Part model, mm, in its own coordinate system. A direction names the side the tool comes from. Coordinates: 2 decimals unless noted, no trailing zeros. Loops run counter-clockwise (first coordinate to the right, second up) from the corner with the lowest first, then second, coordinate; pieces in that order, holes last. Notation, with made-up numbers: M 60,8 L 82,8 A14 ccw 82,31 Z; hole C 78,45.25 d10. An arc over 180 degrees is marked long. Use a Markdown table: item, result. Add a question column.
1) Band-saw the part on A-A (z = 0.3). List the corners of the cut face in (x, y), plus the area to 3 significant figures.
2) Pull direction X, two halves, no side cores. Call faces 4 (the cylindrical face through (2, 3.7, 0.2)), 5 (the cylindrical face through (-6.048, 0.884, 0.85)), 6 (the cylindrical face through (-6.707, 0.627, 0.857)): released by +X, released by -X, zero draft, split by the parting line, or undercut.
3) Tool access for faces 1 (the cylindrical face through (1.95, 3.68, 0.86)), 2 (the cylindrical face through (-6.06, 0.88, 0.14)), 3 (the cylindrical face through (1.26, 3.53, 0.85)): list every direction of +Z, -Z, +X, -X, +Y, -Y with a clear straight run to the whole face (end or side of a thin tool).
4) Wall check: probe 1 along X at (y, z) = (14, 0.6); probe 2 along X at (y, z) = (-14, 0.15); probe 3 along Z at (x, y) = (-11.75, 21). Give the ranges that are in metal, low to high. Write a range as from..to.
Autodesk Inventor part; units mm, degrees
ref_plane "YZ Plane" through (0, 0, 0) normal (1, 0, 0) x (0, 1, 0)
ref_plane "XZ Plane" through (0, 0, 0) normal (0, 1, 0) x (-1, 0, 0)
ref_plane "XY Plane" through (0, 0, 0) normal (0, 0, 1) x (1, 0, 0)
sketch "スケッチ1" plane through (0, 0, 0) normal (0, 0, 1) x (1, 0, 0)
  circle A0 centre (2, -12.5) radius 2.5
  circle A1 centre (-7, 17.5) radius 5
  line L0 (-2.1115, 18.5499) -> (4.4443, -11.9751)
  line L1 (-0.3296, -13.4072) -> (-11.6592, 15.6856)
  arc A2 (-1.1338, 18.7599) -> (-12.591, 15.3227) centre (-7, 17.5) ccw
  arc A3 (-1.2614, -13.7701) -> (5.422, -11.7651) centre (2, -12.5) ccw
  line L2 (-1.1338, 18.7599) -> (5.422, -11.7651)
  line L3 (-1.2614, -13.7701) -> (-12.591, 15.3227)
  point P0 (0, 0)
  dimension "d0" = 1
  dimension "d1" = 1
extrude "押し出し1" add sketch "スケッチ1" along normal blind 1
fillet "フィレット1" radius 0.5 16 edges at (2.7184, -14.8946, 1) (-5.9944, 1.1392, 1) (-8.4367, 22.2891, 1) (1.1664, 3.2874, 1) (-8.7241, 23.247, 1) (-6.9262, 0.7763, 1) (3.0057, -15.8524, 1) (2.1441, 3.4974, 1) (-8.7241, 23.247, 0) (-6.9262, 0.7763, 0) (3.0057, -15.8524, 0) (2.1441, 3.4974, 0) (2.7184, -14.8946, 0) (-5.9944, 1.1392, 0) (-8.4367, 22.2891, 0) (1.1664, 3.2874, 0)
properties part number "Belt"
Entries:
| question | item | result |
|---|---|---|
| 1 | outline | M -12.55,15.34 L -1.22,-13.75 A3.46 ccw 5.38,-11.77 L -1.17,18.75 A5.96 ccw long Z; hole M -11.7,15.67 L -0.37,-13.42 A2.54 ccw 4.49,-11.97 L -2.07,18.56 A5.04 ccw long Z |
| 1 | area | 82.1 mm2 |
| 2 | face 4 | released by +X |
| 2 | face 5 | undercut |
| 2 | face 6 | released by -X |
| 3 | face 1 | +Z, +X, +Y |
| 3 | face 2 | -Z |
| 3 | face 3 | +Z |
| 4 | probe 1 | -12.07..-11.01, -1.12..-0.12 |
| 4 | probe 2 | -1..-0.18, 4.18..5 |
| 4 | probe 3 | 0.2..0.8 |
